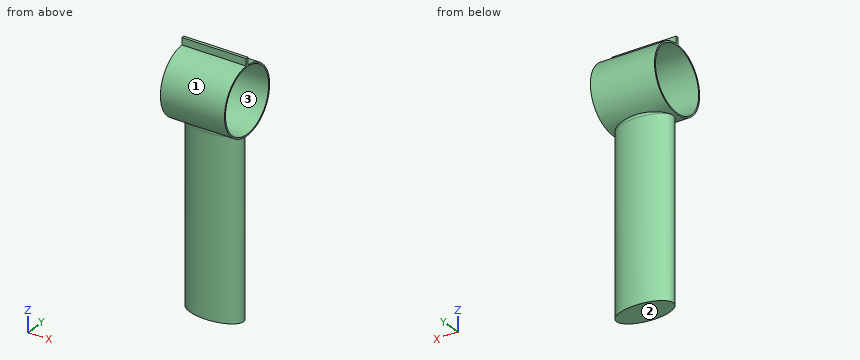
```python
from build123d import *

# Parameters (mm, degrees)
CLASP_SKETCH_R                  = 45
CLASP_EXTRUDE_DEPTH             = 90
SHAFT_EXTRUDE_REACH             = 147.314
SHAFT_EXTRUDE_END_RADIUS        = 47
SHAFT_SKETCH_RX                 = 40
SHAFT_SKETCH_RY                 = 20
SHAFT_EXTRUDE_DIRECTION_2_DEPTH = 250


with BuildPart() as part:
    # Clasp Sketch → Clasp Extrude (new body)
    with BuildSketch(Plane(origin=(0, 0, 0), x_dir=(0, 0, -1), z_dir=(1, 0, 0))):
        with BuildLine():
            Line((-56.957427527, -2), (-56.957427527, 2))
            Line((-56.957427527, 2), (-46.957427527, 2))
            ThreePointArc((-46.957427527, 2), (47, 0), (-46.957427527, -2))
            Line((-46.957427527, -2), (-56.957427527, -2))
        make_face()
        with Locations(Location((0, 0, 0), (0, 0, 180))):
            Circle(CLASP_SKETCH_R, mode=Mode.SUBTRACT)
    extrude(amount=CLASP_EXTRUDE_DEPTH)

    # Shaft Extrude: up to this cylinder (the profile starts outside it)
    shaft_extrude_end = Plane(origin=(45, 0, 0), z_dir=(-1, 0, 0)) * Cylinder(SHAFT_EXTRUDE_END_RADIUS, 389.628, mode=Mode.PRIVATE)
    # Shaft Sketch → Shaft Extrude (add, up to the surface)
    with BuildSketch(Plane(origin=(0, 0, -47), x_dir=(-1, 0, 0), z_dir=(0, 0, -1)), mode=Mode.PRIVATE) as shaft_extrude_sk1:
        with Locations(Location((-45, 0), (0, 0, 0))):
            Ellipse(SHAFT_SKETCH_RX, SHAFT_SKETCH_RY)
    shaft_extrude_tool1 = extrude(shaft_extrude_sk1.sketch, amount=-SHAFT_EXTRUDE_REACH, mode=Mode.PRIVATE) - shaft_extrude_end
    add(shaft_extrude_tool1.solids().sort_by_distance((45, 0, -47))[0])
    add(shaft_extrude_tool1.solids().sort_by_distance((45, 0, -47))[1])

    # Shaft Sketch → Shaft Extrude direction 2 (add)
    with BuildSketch(Plane(origin=(0, 0, -47), x_dir=(-1, 0, 0), z_dir=(0, 0, -1))):
        with Locations(Location((-45, 0), (0, 0, 0))):
            Ellipse(SHAFT_SKETCH_RX, SHAFT_SKETCH_RY)
    extrude(amount=SHAFT_EXTRUDE_DIRECTION_2_DEPTH)


solid = part.part
```
CAD build for the part. Positions are in the model's coordinates, mm. Face numbers are marked on the shaded views. Coordinates: 2 decimals unless noted, no trailing zeros. Order: outer loops, then holes, each group sorted by start corner. A loop starts at its lowest first (then second) coordinate and runs counter-clockwise, first axis right, second up. Notation, with made-up numbers: (84, 17) -> (115, 17) arc R20 ccw to (115, 51) -> close; hole circle Ø5 at (31, 13). An arc over 180 degrees is marked (long way). Use one line per item in the form item = value. Start each with the question number.
1) Band-saw the part on A-A on z = 0. Give the cut face in (x, y).
2) Pull direction Y, two halves, no side cores. Call the marked faces 1, 2 and 3: +Y half, -Y half, draft (parallel to the pull), parting line (faces both ways), or undercut.
3) Drop flat-ended pins along their axis: pin 1 (3 mm diameter, centred on x = 41, z = 53.5, fed in from -Y); pin 2 (6 mm diameter, centred on x = 36, z = -224, fed in from +Y); pin 3 (6 mm diameter, centred on y = -0.5, z = -210.5, fed in from +X). Give the stop position or say it passes through.
4) Band-saw the part on B-B on y = -34. Give the cut face in (x, z).
5) Drill centre lines: L1, parallel to Y at x = 67.5, z = 0; L2, parallel to Z at x = 55.5, y = 2.5; L3, parallel to Z at x = 36, y = 14. Where is each one in solid material? Low to high. Write a range as [from, to].
Entries:
q1.outline = (0, -47) -> (90, -47) -> (90, -45) -> (0, -45) -> close; (0, 45) -> (90, 45) -> (90, 47) -> (0, 47) -> close
q2.face_1 = parting line
q2.face_2 = draft
q2.face_3 = undercut
q3.pin_1 = -2
q3.pin_2 = 19.77
q3.pin_3 = 85
q4.outline = (0, -32.45) -> (90, -32.45) -> (90, -29.48) -> (0, -29.48) -> close; (0, 29.48) -> (90, 29.48) -> (90, 32.45) -> (0, 32.45) -> close
q5.L1 = [-47, -45], [45, 47]
q5.L2 = [-297, -44.93], [44.93, 46.93]
q5.L3 = [-297, -42.77], [42.77, 44.87]
